Source: three-view drawing plus pictorial views. Frame: mm from the lowest corner of the part. A direction names the side the tool comes from. Coordinates: 2 decimals unless noted, no trailing zeros. Order: outer loops, then holes, each group sorted by start corner. A loop starts at its lowest first (then second) coordinate and runs counter-clockwise, first axis right, second up. Notation, with made-up numbers: M 86,51 L 105,51 A28 cw 105,70 Z; hole C 75.25,55 d6. An arc over 180 degrees is marked long. One line per question, with ' | ' between items.
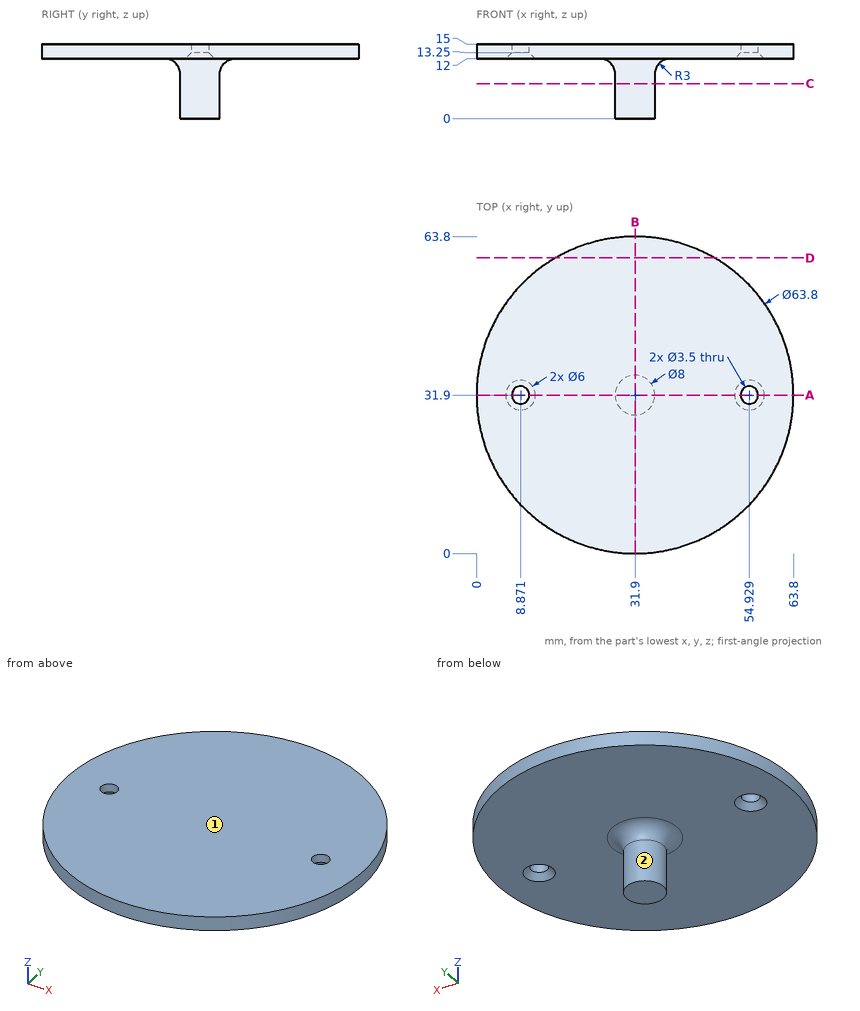
1. Section B-B, the plane x = 31.9. Output: boundary loops of the cut face in (y, z).
Response values:
outline: M 0,12 L 24.9,12 A3 cw 27.9,9 L 27.9,0 L 35.9,0 L 35.9,9 A3 cw 38.9,12 L 63.8,12 L 63.8,15 L 0,15 Z
2. Section D-D, the plane y = 59.5. Output: boundary loops of the cut face in (x, z).
Response values:
outline: M 15.9,12 L 47.9,12 L 47.9,15 L 15.9,15 Z
3. Section C-C, the plane z = 7. Output: boundary loops of the cut face in (x, y).
Response values:
outline: C 31.9,31.9 d8
4. Access query for the marked faces 1 and 2. Directions: +Z, -Z, +X, -X, +Y, -Y. A direction counts if a zero-diameter tool reaches every point of the face in a straight line with its end or side. Return the directions, or none.
Response values:
face 1: +Z, +X, -X, +Y, -Y | face 2: -Z
5. Section A-A, the plane y = 31.9. Output: boundary loops of the cut face in (x, z).
Response values:
outline: M 0,12 L 5.87,12 L 7.12,13.25 L 7.12,15 L 0,15 Z; M 10.62,13.25 L 11.87,12 L 24.9,12 A3 cw 27.9,9 L 27.9,0 L 35.9,0 L 35.9,9 A3 cw 38.9,12 L 51.93,12 L 53.18,13.25 L 53.18,15 L 10.62,15 Z; M 56.68,13.25 L 57.93,12 L 63.8,12 L 63.8,15 L 56.68,15 Z
6. Material intervals for line 1 (X direction, y = 32, z = 13.5); line 2 (Z direction, x = 32, y = 40); line 3 (X direction, y = 33.5, z = 5.75), sorted ascending. Write a range as [from, to].
Response values:
line 1: x = [0, 7.12], [10.62, 53.18], [56.68, 63.8] | line 2: z = [12, 15] | line 3: x = [28.23, 35.57]
7. Pin query (flat end, axial travel): P1, Ø4.5, axis at x = 8.871, y = 31.9, coming from the -Z side; P2, Ø4, axis at x = 54.929, y = 31.9, coming from the -Z side; P3, Ø5, axis at y = 38, z = 9, coming from the +X side; P4, Ø8, axis at x = 20.5, z = 6.5, coming from the -Y side. Return the tip coordinate at first contact, or that it passes through.
Response values:
P1: stops at z = 12.75 | P2: stops at z = 13 | P3: stops at x = 33.64 | P4: passes through
